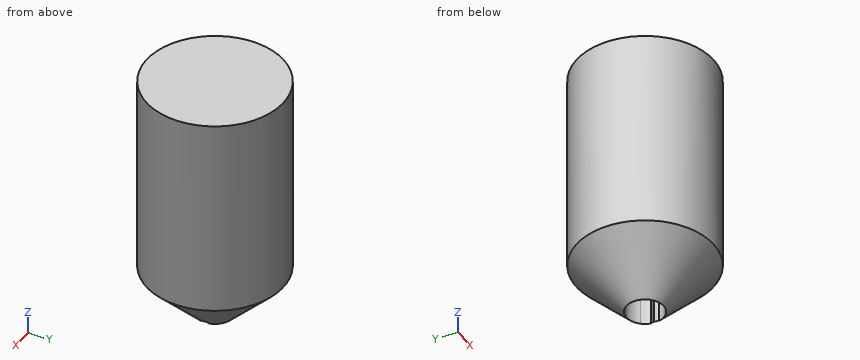
```python
from build123d import *
from build123d import SkipClean  # not in build123d's __all__

# Parameters (mm, degrees)
F0_R       = 34.8665776849
F1_DEPTH   = 127
F2_SIZE    = 25.4
F3_W       = 0.0296507081
F3_H       = 2.1137676667
F3_W_2     = 1.5040034195
F3_H_2     = 6.3516600603
F3_W_3     = 5.515434417
F1_FACE_R  = 9.4665776849
F1_FACE1_R = 34.8665776849
F4_DEPTH   = 76.2


with BuildPart() as f1:
    # F0 (on Top) → F1 (new body)
    with BuildSketch(Plane.XY):
        Circle(F0_R)
    extrude(amount=F1_DEPTH)

    # F2
    f2_edges = [f1.edges().sort_by_distance(p)[0] for p in [
        (-34.866578, 0, 0),
    ]]
    chamfer(f2_edges, length=F2_SIZE)

    # F3 (on face) + F1_face (on face) + F1_face1 (on face) → F4 (cut)
    with BuildSketch(Plane(origin=(0, 0, 0), x_dir=(1, 0, 0), z_dir=(0, 0, -1))):
        with Locations((7.0046124826, 1.0568838334)):
            Rectangle(F3_W, F3_H)
        with Locations((7.0046124826, -1.0568838334)):
            Rectangle(F3_W, F3_H)
        with Locations((0.7520017098, -3.1758300302)):
            Rectangle(F3_W_2, F3_H_2)
        with BuildLine():
            Line((7.0194378366, 2.1137676667), (7.0194378366, 0))
            Line((7.0194378366, 0), (9.4665776849, 0))
            ThreePointArc((9.4665776849, 0), (9.4066364158, 1.0636185423), (9.2275716911, 2.1137676667))
            Line((9.2275716911, 2.1137676667), (7.0194378366, 2.1137676667))
        make_face()
        with BuildLine():
            Line((7.0194378366, 0), (7.0194378366, -2.1137676667))
            Line((7.0194378366, -2.1137676667), (9.2275716911, -2.1137676667))
            ThreePointArc((9.2275716911, -2.1137676667), (9.4066364158, -1.0636185423), (9.4665776849, 0))
            Line((9.4665776849, 0), (7.0194378366, 0))
        make_face()
        with BuildLine():
            ThreePointArc((9.4665776849, 0), (9.4066364158, -1.0636185423), (9.2275716911, -2.1137676667))
            Line((9.2275716911, -2.1137676667), (11.9433682412, -2.1137676667))
            Line((11.9433682412, -2.1137676667), (11.9433682412, 2.1137676667))
            Line((11.9433682412, 2.1137676667), (9.2275716911, 2.1137676667))
            ThreePointArc((9.2275716911, 2.1137676667), (9.4066364158, 1.0636185423), (9.4665776849, 0))
        make_face()
        with Locations((-4.2617206281, 3.1758300302)):
            Rectangle(F3_W_3, F3_H_2)
        with Locations((-4.2617206281, -3.1758300302)):
            Rectangle(F3_W_3, F3_H_2)
        Polygon((1.5040034195, -6.3516600603), (7.0194378366, -6.3516600603), (7.0194378366, -2.1137676667), (6.9897871285, -2.1137676667), (6.9897871285, 0), (1.5040034195, 0), align=None)
        Polygon((1.5040034195, 6.3516600603), (1.5040034195, 0), (6.9897871285, 0), (6.9897871285, 2.1137676667), (7.0194378366, 2.1137676667), (7.0194378366, 6.3516600603), align=None)
        with Locations((0.7520017098, 3.1758300302)):
            Rectangle(F3_W_2, F3_H_2)
        with Locations((-0.7520017098, 3.1758300302)):
            Rectangle(F3_W_2, F3_H_2)
        with BuildLine():
            Line((-1.5040034195, 6.3516600603), (0, 6.3516600603))
            Line((0, 6.3516600603), (0, 9.4665776849))
            ThreePointArc((0, 9.4665776849), (-3.8397662477, 8.6528774535), (-7.0194378366, 6.3516600603))
            Line((-7.0194378366, 6.3516600603), (-1.5040034195, 6.3516600603))
        make_face()
        with Locations((-0.7520017098, -3.1758300302)):
            Rectangle(F3_W_2, F3_H_2)
        with BuildLine():
            Line((0, 9.4665776849), (0, 6.3516600603))
            Line((0, 6.3516600603), (1.5040034195, 6.3516600603))
            Line((1.5040034195, 6.3516600603), (7.0194378366, 6.3516600603))
            ThreePointArc((7.0194378366, 6.3516600603), (3.8397662477, 8.6528774535), (0, 9.4665776849))
        make_face()
        with BuildLine():
            Line((0, -6.3516600603), (0, -9.4665776849))
            ThreePointArc((0, -9.4665776849), (3.8397662477, -8.6528774535), (7.0194378366, -6.3516600603))
            Line((7.0194378366, -6.3516600603), (1.5040034195, -6.3516600603))
            Line((1.5040034195, -6.3516600603), (0, -6.3516600603))
        make_face()
    with BuildSketch(Plane(origin=(0, 0, 0), x_dir=(1, 0, 0), z_dir=(0, 0, -1))):
        Circle(F1_FACE_R)
    with BuildSketch(Plane.XY.offset(127)):
        Circle(F1_FACE1_R)
    extrude(amount=-F4_DEPTH, dir=(0, 0, -1), mode=Mode.SUBTRACT)

    # F5: F1 across plane


with BuildPart() as f1_1:
    add(f1.part, clean=False)
    with SkipClean():  # cleaning this boolean's faces spoils the solid; the shape is the same uncleaned
        add(f1.part.mirror(Plane.XZ), clean=False)


solid = f1_1.part
```
Could you check a few things on this model? Use its own coordinates, in mm. Coordinates: 2 decimals unless noted, no trailing zeros. Loops run counter-clockwise (first coordinate to the right, second up) from the corner with the lowest first, then second, coordinate; pieces in that order, holes last.
1) Imagine slicing it at C-C (z = 107.5). List the corners of the cut face in (x, y) for me.
Reported:
outline: circle Ø69.73 at (0, 0)
2) Imagine slicing it at A-A (z = 68). List the corners of the cut face in (x, y) for me, and give its area (3 significant figures).
Reported:
outline: circle Ø69.73 at (0, 0); hole (9.23, -2.11) - (11.94, -2.11) - (11.94, 2.11) - (9.23, 2.11) arc R9.47 ccw (long way) to start
area: 3,530 mm2
3) Will these pins go through, and if not, where does the flat tip stop? pin 1 Ø3 at (y, z) = (-2.5, 51.5) entering from -X; pin 2 Ø1 at (x, z) = (10.5, 98) entering from -Y; pin 3 Ø1 at (x, z) = (-9, 43.5) entering from +Y.
Reported:
pin 1: stops at x = -34.85
pin 2: stops at y = -33.4
pin 3: stops at y = 33.81
4) Please list where these lines run through material, in increasing order: line 1 along X through (y, z) = (4, 33); line 2 along Z through (x, y) = (17, -13); line 3 along X through (y, z) = (-2, 55).
Reported:
line 1: x = -34.64 to -8.58, 8.58 to 34.64
line 2: z = 11.93 to 127
line 3: x = -34.81 to -9.25, 11.94 to 34.81
5) Imagine slicing it at B-B (y = 0). List the corners of the cut face in (x, z) for me.
Reported:
outline: (-34.87, 25.4) - (-9.47, 0) - (-9.47, 76.2) - (11.94, 76.2) - (11.94, 2.48) - (34.87, 25.4) - (34.87, 127) - (-34.87, 127) - close
